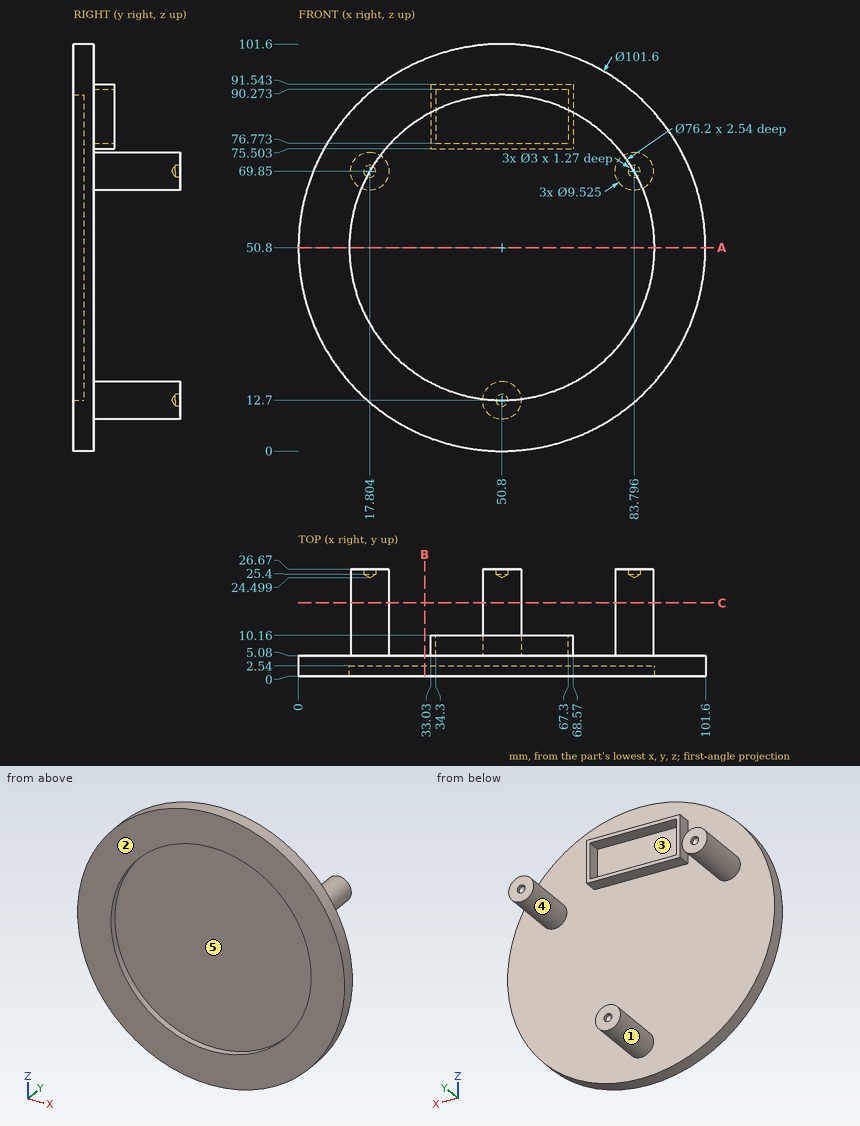
Answer from the drawing. Dimensions are ordinates in mm from the lowest x, y and z of the part. A direction names the side the tool comes from. Give positions to 0.01 mm unless a question says otherwise; leave off trailing zeros. Write each loop counter-clockwise with the first axis right and the second up, starting at its lowest first coordinate (ties: lowest second). Pieces come first, ordered by that corner, then holes. Notation, with made-up numbers: (55, 28) -> (78, 28) arc R10 cw to (78, 35) -> close; hole circle Ø11 at (47.25, 56). An arc over 180 degrees is marked (long way). Use a Markdown table: item, result.
(1) Section C-C, the plane y = 18.25 is taken. Give the number of separate pieces and of enclosed holes in the cut face, then the cut area to 3 significant figures.
Return value:
| item | result |
|---|---|
| separate pieces | 3 |
| enclosed holes | 0 |
| area | 214 mm2 |
(2) Find the intervals of material crossed by probe 1 along X at (y, z) = (26.1, 69.85) (1 decimal); probe 2 along X at (y, z) = (25.8, 12.7); probe 3 along Y at (x, z) = (82, 88.5), in increasing order. Write a range as from..to.
Return value:
| item | result |
|---|---|
| probe 1 | 13..16.3, 19.3..22.6, 79..82.3, 85.3..88.6 |
| probe 2 | 46.04..49.3, 52.3..55.56 |
| probe 3 | 0..5.08 |
(3) Section B-B, the plane x = 31.5 is taken. Determine the outline of the cut face in (y, z).
Return value:
| item | result |
|---|---|
| outline | (0, 3.81) -> (5.08, 3.81) -> (5.08, 97.79) -> (0, 97.79) -> (0, 83.65) -> (2.54, 83.65) -> (2.54, 17.95) -> (0, 17.95) -> close |
(4) Section A-A, the plane z = 50.8 is taken. Determine the outline of the cut face in (x, y).
Return value:
| item | result |
|---|---|
| outline | (0, 0) -> (12.7, 0) -> (12.7, 2.54) -> (88.9, 2.54) -> (88.9, 0) -> (101.6, 0) -> (101.6, 5.08) -> (0, 5.08) -> close |
(5) Determine the mould class of the marked faces 1, 2 and 3 for opening direction X: released by +X, released by -X, zero draft, split by the parting line, or undercut.
Return value:
| item | result |
|---|---|
| face 1 | split by the parting line |
| face 2 | zero draft |
| face 3 | undercut |
(6) For the marked faces 4 and 5, determine the directions among +Z, -Z, +X, -X, +Y, -Y from which every point of the face is accessible in a straight line to the end or side of a thin tool.
Return value:
| item | result |
|---|---|
| face 4 | +Y |
| face 5 | -Y |
(7) Flat-ended cylindrical pins translate along their axes: P1, Ø1, axis at x = 67, z = 75, coming from the -Y side; P2, Ø13, axis at x = 53.5, z = 82, coming from the +Y side; P3, Ø1.5, axis at x = 54.5, y = 7, coming from the +Z side; P4, Ø8, axis at y = 19, z = 25, coming from the -X side. Find the tip coordinate at first contact, or state that the pin passes through.
Return value:
| item | result |
|---|---|
| P1 | y = 2.54 |
| P2 | y = 10.16 |
| P3 | z = 91.54 |
| P4 | through |
